from build123d import *

# Parameters (mm, degrees)
F1_DEPTH = 300
F2_R     = 3.25
F3_DEPTH = 25
F5_DEPTH = 4
F8_DEPTH = 4


with BuildPart() as f1:
    # F0 (on Right) → F1 (new body)
    with BuildSketch(Plane.YZ):
        Polygon((0, 90), (0, 0), (80, 0), (80, 4), (4, 4), (4, 90), align=None)
    extrude(amount=F1_DEPTH)

    # F2 (on face) → F3 (cut)
    with BuildSketch(Plane.XY.offset(4)):
        with Locations((20, 42)):
            Circle(F2_R)
        with Locations((280, 42)):
            Circle(F2_R)
    extrude(amount=-F3_DEPTH, mode=Mode.SUBTRACT)

    # F4 (on Right) → F5 (join)
    with BuildSketch(Plane.YZ):
        Polygon((4, 4), (80, 4), (4, 90), align=None)
    extrude(amount=F5_DEPTH)

    # F7 (on offset) → F8 (join)
    with BuildSketch(Plane.YZ.offset(300)):
        Polygon((80, 4), (4, 90), (4, 4), align=None)
    extrude(amount=-F8_DEPTH)


solid = f1.part
Source: CAD feature listing. Evaluate the final solid. Frame: model axes, mm. A direction names the side the tool comes from. Round coordinates to 2 decimals unless told otherwise and drop trailing zeros. Order: outer loops, then holes, each group sorted by start corner. A loop starts at its lowest first (then second) coordinate and runs counter-clockwise, first axis right, second up. Notation, with made-up numbers: (84, 77.25) -> (100, 77.25) arc R19 ccw to (100, 110.25) -> close; hole circle Ø2 at (21, 22.25). An arc over 180 degrees is marked (long way). Answer as CSV lines item,"result".
Item 1: Line query: L1, parallel to Y at x = 280, z = 2.4; L2, parallel to X at y = 20, z = 24; L3, parallel to Z at x = 156, y = 34. Output: solid intervals per line, ascending.
A:
L1,"0 to 38.75, 45.25 to 80"
L2,"0 to 4, 296 to 300"
L3,"0 to 4"
Item 2: Pull-direction query (X, two-part tool) for faces 3 (the face through (148, 39, 0)), 4 (the face through (0, 31, 36)), 5 (the face through (148, 43, 4)), 6 (the face through (300, 31, 36)); classes: pulls with the +X half, pulls with the -X half, needs draft (parallel to the pull), parting line crosses it, or undercut.
A:
face 3,"needs draft"
face 4,"pulls with the -X half"
face 5,"undercut"
face 6,"pulls with the +X half"
Item 3: Reachability of faces 1 (the face through (148, 4, 46)), 2 (the face through (1.97, 42.53, 46.4)) from +Z, -Z, +X, -X, +Y, -Y: full face, straight path, thin tool, end or side. Return the list, or none.
A:
face 1,"+Z, +Y"
face 2,"+Z, +X, -X, +Y"
Item 4: Section B-B, the plane x = 20. Return loops of the section in (y, z), plus the area to 3 significant figures.
A:
outline,"(0, 0) -> (38.75, 0) -> (38.75, 4) -> (4, 4) -> (4, 90) -> (0, 90) -> close; (45.25, 0) -> (80, 0) -> (80, 4) -> (45.25, 4) -> close"
area,"638 mm²"
Item 5: Section A-A, the plane y = 42. Return loops of the section in (x, z), plus the area to 3 significant figures.
A:
outline,"(0, 0) -> (16.75, 0) -> (16.75, 4) -> (4, 4) -> (4, 47) -> (0, 47) -> close; (23.25, 0) -> (276.75, 0) -> (276.75, 4) -> (23.25, 4) -> close; (283.25, 0) -> (300, 0) -> (300, 47) -> (296, 47) -> (296, 4) -> (283.25, 4) -> close"
area,"1,490 mm²"
Item 6: Pin query (flat end, axial travel): pin 1 Ø4 at (x, y) = (242.5, 53.5) entering from +Z; pin 2 Ø12 at (y, z) = (20.5, 67.5) entering from -X. Return the tip coordinate at first contact, or that it passes through.
A:
pin 1,"z = 4"
pin 2,"x = 0"
Item 7: Section D-D, the plane z = 72.5. Return loops of the section in (x, y), plus the area to 3 significant figures.
A:
outline,"(0, 0) -> (300, 0) -> (300, 19.47) -> (296, 19.47) -> (296, 4) -> (4, 4) -> (4, 19.47) -> (0, 19.47) -> close"
area,"1,320 mm²"
Item 8: Section C-C, the plane y = 13.5. Return loops of the section in (x, z), plus the area to 3 significant figures.
A:
outline,"(0, 0) -> (300, 0) -> (300, 79.25) -> (296, 79.25) -> (296, 4) -> (4, 4) -> (4, 79.25) -> (0, 79.25) -> close"
area,"1,800 mm²"
